```python
from build123d import *

# Parameters (mm, degrees)
SKETCH1_W           = 6
SKETCH1_H           = 3
TAPPED_HOLE1_REACH  = 18.763
TAPPED_HOLE1_BORE_R = 1.65
CIRPATTERN1_COUNT   = 2
CIRPATTERN1_ANGLE   = 90
CHAMFER1_SIZE       = 0.2


with BuildPart() as part:
    # Sketch1 → Revolve1 (revolve)
    with BuildSketch(Plane(origin=(0, 0, 0), x_dir=(0, 0, -1), z_dir=(1, 0, 0)), mode=Mode.PRIVATE) as revolve1_sk:
        with Locations((3, 5.5)):
            Rectangle(SKETCH1_W, SKETCH1_H)
    revolve(revolve1_sk.sketch.rotate(Axis((0, 0, 0), (0, 0, -1)), 90), axis=Axis((0, 0, 0), (0, 0, -1)))

    # Tapped Hole1 bore → Tapped Hole1 (cut, up to next)
    with BuildSketch(Plane(origin=(0, 7, 0), x_dir=(1, 0, 0), z_dir=(0, 1, 0)), mode=Mode.PRIVATE) as tapped_hole1_sk1:
        with Locations((0, 3)):
            Circle(TAPPED_HOLE1_BORE_R)
    tapped_hole1_tool1 = extrude(tapped_hole1_sk1.sketch, amount=-TAPPED_HOLE1_REACH, mode=Mode.PRIVATE) & part.part
    tapped_hole1 = tapped_hole1_tool1.solids().sort_by_distance((0, 7, -3))[0]
    add(tapped_hole1, mode=Mode.SUBTRACT)

    # CirPattern1: Tapped Hole1 ×2 about axis
    cirpattern1_axis = Axis((0, 0, 0), (0, 0, -1))
    for i in range(1, CIRPATTERN1_COUNT):
        add(tapped_hole1.rotate(cirpattern1_axis, i * CIRPATTERN1_ANGLE / (CIRPATTERN1_COUNT - 1)), mode=Mode.SUBTRACT)

    # Chamfer1
    chamfer1_edges = [part.edges().sort_by_distance(p)[0] for p in [
        (-4, 0, -6),
        (-4, 0, 0),
        (-7, 0, -6),
    ]]
    chamfer(chamfer1_edges, length=CHAMFER1_SIZE)

    # Sketch4 → Cut-Revolve1 (revolve, cut)
    with BuildSketch(Plane(origin=(0, 0, 0), x_dir=(0, 0, -1), z_dir=(1, 0, 0)), mode=Mode.PRIVATE) as cut_revolve1_sk:
        Polygon((0.577350269, 7), (0, 6), (0, 7), align=None)
    revolve(cut_revolve1_sk.sketch.rotate(Axis((0, 0, 0), (0, 0, -1)), 90), axis=Axis((0, 0, 0), (0, 0, -1)), mode=Mode.SUBTRACT)


solid = part.part
```
The model under review builds one solid part; all positions refer to its coordinate system, in mm. A direction names the side the tool comes from. Round coordinates to 2 decimals unless told otherwise and drop trailing zeros. Loops run counter-clockwise (first coordinate to the right, second up) from the corner with the lowest first, then second, coordinate; pieces in that order, holes last. Notation, with made-up numbers: (-5, -29) - (23, -29) arc R19 ccw to (23, 2) - close; hole circle Ø9 at (12, 64.5). An arc over 180 degrees is marked (long way). Use a Markdown table: item, result. Add a question column.
Q1. For probe 1 along Y at (x, z) = (0, -2.45); probe 2 along X at (y, z) = (1.5, -5.3), list the stretches that pass through material, from the lowest coordinate up.
Q2. Machinability: for faces 1 (the face through (5.35, 1.65, -3.07)), 2 (the face through (0.1, 4.4, -6)), which of the approach directions +Z, -Z, +X, -X, +Y, -Y give a long, thin tool a straight path to every point of the face, cutting with its end or side? Answer none if there is none.
Q3. Add section C-C (z = -3). State the section outline as (x, y) points.
Q4. Insertion check: pin 1 Ø1 at (y, z) = (2.5, -3.5) entering from -X; pin 2 Ø1.5 at (x, z) = (3, -1.5) entering from -Y; pin 3 Ø1 at (y, z) = (3, -1.5) entering from -X. Each pin has a flat end and moves straight along its axis. Give the tip position at first contact, or say it passes through.
Q5. Add section A-A (x = 0). State the section outline as (y, z) points.
Q6. The part is to be moulded in two halves that separate along Y. For faces 3 (the face through (-2.95, -2.7, -3.04)), 4 (the face through (-1.65, 5.35, -3.07)), 5 (the face through (3.763, -5.902, -3.225)), say which applies: pulls with the +Y half, pulls with the -Y half, needs draft (parallel to the pull), parting line crosses it, or undercut.
Worked answers:
| question | item | result |
|---|---|---|
| 1 | probe 1 | -7 to -4 |
| 1 | probe 2 | -6.84 to -3.71, 3.71 to 6.84 |
| 2 | face 1 | +X |
| 2 | face 2 | -Z, +X, -X, +Y, -Y |
| 3 | outline | (-1.65, 3.64) - (-1.65, 6.8) arc R7 ccw (long way) to (6.8, -1.65) - (3.64, -1.65) arc R4 cw (long way) to start; (1.65, 3.64) arc R4 cw to (3.64, 1.65) - (6.8, 1.65) arc R7 ccw to (1.65, 6.8) - close |
| 4 | pin 1 | x = -6.71 |
| 4 | pin 2 | y = -6.63 |
| 4 | pin 3 | x = -6.54 |
| 5 | outline | (-7, -5.8) - (-6.8, -6) - (-4.2, -6) - (-4, -5.8) - (-4, -0.2) - (-4.2, 0) - (-6, 0) - (-7, -0.58) - close; (4, -5.8) - (4.2, -6) - (6.8, -6) - (7, -5.8) - (7, -4.65) - (4, -4.65) - close; (4, -1.35) - (7, -1.35) - (7, -0.58) - (6, 0) - (4.2, 0) - (4, -0.2) - close |
| 6 | face 3 | undercut |
| 6 | face 4 | needs draft |
| 6 | face 5 | parting line crosses it |
